from build123d import *

# Parameters (mm, degrees)
SKETCH_1_W          = 160
SKETCH_1_H          = 80
EXTRUDE_1_DEPTH     = 8
SKETCH_2_W          = 150
SKETCH_2_H          = 75
CUT_EXTRUDE_1_DEPTH = 6
SKETCH_3_W          = 15
SKETCH_3_H          = 10
CUT_EXTRUDE_2_DEPTH = 90.799777283


with BuildPart() as part:
    # 草图1 → 凸台-拉伸1 (new body)
    with BuildSketch(Plane.XY):
        Rectangle(SKETCH_1_W, SKETCH_1_H)
    extrude(amount=EXTRUDE_1_DEPTH)

    # 草图2 → 切除-拉伸1 (cut)
    with BuildSketch(Plane(origin=(0, 40, 0), x_dir=(1, 0, 0), z_dir=(0, 1, 0))):
        Rectangle(SKETCH_2_W, SKETCH_2_H)
    extrude(amount=-CUT_EXTRUDE_1_DEPTH, mode=Mode.SUBTRACT)

    # 草图3 → 切除-拉伸2 (cut, through all)
    with BuildSketch(Plane.XY.offset(8)):
        with Locations((50, 0)):
            Rectangle(SKETCH_3_W, SKETCH_3_H)
    extrude(amount=-CUT_EXTRUDE_2_DEPTH, mode=Mode.SUBTRACT)


solid = part.part
Here's how the part is built. I have some questions about the finished solid (model axes, mm). A direction names the side the tool comes from. Round coordinates to 2 decimals unless told otherwise and drop trailing zeros. Order: outer loops, then holes, each group sorted by start corner. A loop starts at its lowest first (then second) coordinate and runs counter-clockwise, first axis right, second up. Notation, with made-up numbers: (81, 24) -> (129, 24) arc R9 cw to (129, 39) -> close; hole circle Ø5 at (43.25, -6). An arc over 180 degrees is marked (long way). Use CSV: the item, a comma, the result in double quotes.
1. Thinking about a two-plate mould opening in X: for faces 4 (the face through (80, -1, 4)), 5 (the face through (77, 40, 4)), 6 (the face through (50, 5, 4)), which applies, pulls with the +X half, pulls with the -X half, needs draft (parallel to the pull), parting line crosses it, or undercut?
Recorded:
face 4,"pulls with the +X half"
face 5,"needs draft"
face 6,"undercut"
2. I'm going to push a flat-ended pin straight in: P1, Ø4, axis at x = 49.5, z = 3, coming from the +Y side. Where does the tip first touch, or does it pass through?
Recorded:
P1,"stops at y = 34"
3. I need wall thicknesses on line 1 along X through (y, z) = (-3.5, 5.75); line 2 along Y through (x, z) = (12, 4); line 3 along X through (y, z) = (35, 2.25). Which ranges of each line are inside material? Lowest first, please.
Recorded:
line 1,"x = -80 to 42.5, 57.5 to 80"
line 2,"y = -40 to 34"
line 3,"x = -80 to -75, 75 to 80"
4. I want a section at B-B on z = 4. List the corners of the cut face in (x, y) for me.
Recorded:
outline,"(-80, -40) -> (80, -40) -> (80, 40) -> (75, 40) -> (75, 34) -> (-75, 34) -> (-75, 40) -> (-80, 40) -> close; hole (42.5, -5) -> (57.5, -5) -> (57.5, 5) -> (42.5, 5) -> close"
5. I want a section at C-C on x = -30. List the corners of the cut face in (y, z) for me, and give its area (3 significant figures).
Recorded:
outline,"(-40, 0) -> (34, 0) -> (34, 8) -> (-40, 8) -> close"
area,"592 mm2"
6. Which directions (+Z, -Z, +X, -X, +Y, -Y) give clear straight access to the entire face, cutting with the end or side of a thin tool? Please do faces 1 (the face through (75, 37, 4)), 2 (the face through (57.5, 0, 4)), 3 (the face through (-78, 40, 4)).
Recorded:
face 1,"+Z, -Z, +Y"
face 2,"+Z, -Z"
face 3,"+Z, -Z, +X, -X, +Y"
7. I want a section at A-A on y = 3. List the corners of the cut face in (x, z) for me.
Recorded:
outline,"(-80, 0) -> (42.5, 0) -> (42.5, 8) -> (-80, 8) -> close; (57.5, 0) -> (80, 0) -> (80, 8) -> (57.5, 8) -> close"
